Verification items for the finished model (mm, model axes). Face numbers are marked on the shaded views. A direction names the side the tool comes from. Give positions to 0.01 mm unless a question says otherwise; leave off trailing zeros. Write each loop counter-clockwise with the first axis right and the second up, starting at its lowest first coordinate (ties: lowest second). Pieces come first, ordered by that corner, then holes. Notation, with made-up numbers: (22.5, -25.75) -> (68.5, -25.75) arc R37 cw to (68.5, 10.25) -> close; hole circle Ø8 at (25.5, -20). An arc over 180 degrees is marked (long way). Answer as CSV lines item,"result".
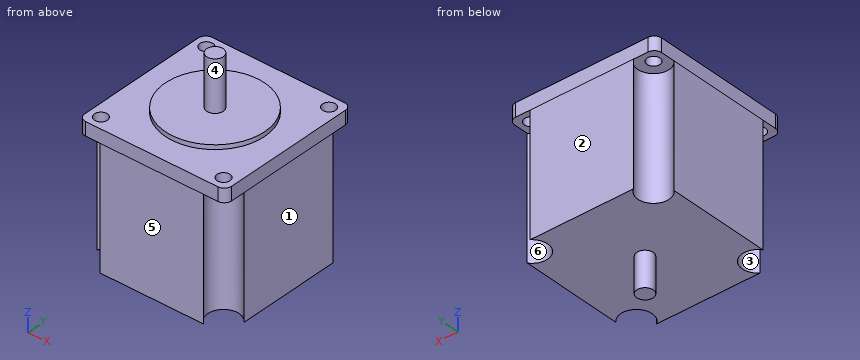
Solid Edge part; units mm, degrees
sketch "Sketch1" plane through (0, 0, 0) normal (0, 0, 1) x (1, 0, 0)
  circle A0 centre (0, 0) radius 3.15
extrude "Protrusion1" add sketch "Sketch1" against normal blind 9
sketch "Sketch2" plane through (0, 0, -9) normal (0, 0, -1) x (1, 0, 0)
  circle A0 centre (0, 0) radius 3.15
extrude "ExtrudedProtrusion_2" add sketch "Sketch2" along normal blind 10.4
sketch "Sketch3" plane through (0, 0, -19.4) normal (0, 0, -1) x (1, 0, 0)
  circle A0 centre (0, 0) radius 19.05
extrude "ExtrudedProtrusion_3" add sketch "Sketch3" along normal blind 1.7
sketch "Sketch4" plane through (0, 0, -21.1) normal (0, 0, -1) x (1, 0, 0)
  circle A0 centre (23.55, 23.55) radius 2.5
  circle A1 centre (23.55, -23.55) radius 2.5
  circle A2 centre (-23.55, -23.55) radius 2.5
  circle A3 centre (-23.55, 23.55) radius 2.5
  line L0 (-25.4, -28.2) -> (25.4, -28.2)
  arc A4 (28.2, -25.4) -> (25.4, -28.2) centre (25.4, -25.4) cw
  line L1 (28.2, -25.4) -> (28.2, 25.4)
  arc A5 (25.4, 28.2) -> (28.2, 25.4) centre (25.4, 25.4) cw
  line L2 (25.4, 28.2) -> (-25.4, 28.2)
  arc A6 (-28.2, 25.4) -> (-25.4, 28.2) centre (-25.4, 25.4) cw
  line L3 (-28.2, 25.4) -> (-28.2, -25.4)
  arc A7 (-25.4, -28.2) -> (-28.2, -25.4) centre (-25.4, -25.4) cw
extrude "ExtrudedProtrusion_4" add sketch "Sketch4" along normal blind 5.2
sketch "Sketch5" plane through (0, 0, -26.3) normal (0, 0, -1) x (0, -1, 0)
  line L0 (-28.2, 19.8235) -> (-28.2, -19.8235)
  line L1 (-19.8235, -28.2) -> (19.8235, -28.2)
  line L2 (28.2, -19.8235) -> (28.2, 19.8235)
  line L3 (19.8235, 28.2) -> (-19.8235, 28.2)
  arc A0 (-28.2, -19.8235) -> (-19.8235, -28.2) centre (-23.3345, -23.3345) cw
  arc A1 (19.8235, -28.2) -> (28.2, -19.8235) centre (23.3345, -23.3345) cw
  arc A2 (28.2, 19.8235) -> (19.8235, 28.2) centre (23.3345, 23.3345) cw
  arc A3 (-19.8235, 28.2) -> (-28.2, 19.8235) centre (-23.3345, 23.3345) cw
extrude "ExtrudedProtrusion_5" add sketch "Sketch5" along normal blind 46.1
sketch "Sketch6" plane through (0, 0, -72.4) normal (0, 0, -1) x (-1, 0, 0)
  circle A0 centre (0, 0) radius 3.15
extrude "ExtrudedProtrusion_6" add sketch "Sketch6" along normal blind 13.3
properties material "Stainless steel"
1) Draft check along Y on the marked faces 1, 2 and 3. Enter one of: +Y half, -Y half, draft (parallel to the pull), parting line (faces both ways), or undercut.
Reported:
face 1,"draft"
face 2,"+Y half"
face 3,"undercut"
2) Tool access check on the marked faces 4, 5 and 6. Record the directions out of +Z, -Z, +X, -X, +Y, -Y that give a thin tool (end or side, any length) a straight path to the whole face; none if there is none.
Reported:
face 4,"+Z"
face 5,"+Z, -Z, +X, -X, -Y"
face 6,"-Z"
3) Scan lines: line 1 along X through (y, z) = (23.55, -24.05); line 2 along Y through (x, z) = (23, -24); line 3 along Z through (x, y) = (13, 23). Record each from-to range of solid material in increasing order.
Reported:
line 1,"-28.2 to -26.05, -21.05 to 21.05, 26.05 to 28.2"
line 2,"-28.2 to -25.99, -21.11 to 21.11, 25.99 to 28.2"
line 3,"-72.4 to -21.1"
4) Section check A-A (y = -23.55). Record the boundary of the cut face in (x, z).
Reported:
outline,"(-28.2, -26.3) -> (-26.05, -26.3) -> (-26.05, -21.1) -> (-28.2, -21.1) -> close; (-21.05, -26.3) -> (-17.34, -26.3) -> (-17.34, -72.4) -> (17.34, -72.4) -> (17.34, -26.3) -> (21.05, -26.3) -> (21.05, -21.1) -> (-21.05, -21.1) -> close; (26.05, -26.3) -> (28.2, -26.3) -> (28.2, -21.1) -> (26.05, -21.1) -> close"
5) Depth check by flat-ended pin: pin 1 (6 mm diameter, centred on y = 0.5, z = -73, fed in from +X); pin 2 (4 mm diameter, centred on x = -23.55, y = -23.55, fed in from -Z); pin 3 (9.5 mm diameter, centred on x = -23.33, y = 23.33, fed in from -Z); pin 4 (5 mm diameter, centred on x = -16, y = -15.5, fed in from -Z). Enter the tip coordinate at first touch or a pass-through.
Reported:
pin 1,"x = 28.2"
pin 2,"through"
pin 3,"z = -26.3"
pin 4,"z = -72.4"
6) Section check D-D (z = -46). Record the boundary of the cut face in (x, y).
Reported:
outline,"(-28.2, -19.82) arc R6 cw (long way) to (-19.82, -28.2) -> (19.82, -28.2) arc R6 cw (long way) to (28.2, -19.82) -> (28.2, 19.82) arc R6 cw (long way) to (19.82, 28.2) -> (-19.82, 28.2) arc R6 cw (long way) to (-28.2, 19.82) -> close"
